The model under review builds one solid part; all positions refer to its coordinate system, in mm. Coordinates: 2 decimals unless noted, no trailing zeros. Write each loop counter-clockwise with the first axis right and the second up, starting at its lowest first coordinate (ties: lowest second). Pieces come first, ordered by that corner, then holes. Notation, with made-up numbers: (41, -11) -> (69, -11) arc R12 ccw to (69, 11) -> close; hole circle Ø11 at (76, -21). An arc over 180 degrees is marked (long way). Put each result on its own line as item: value. Start each with the question number.
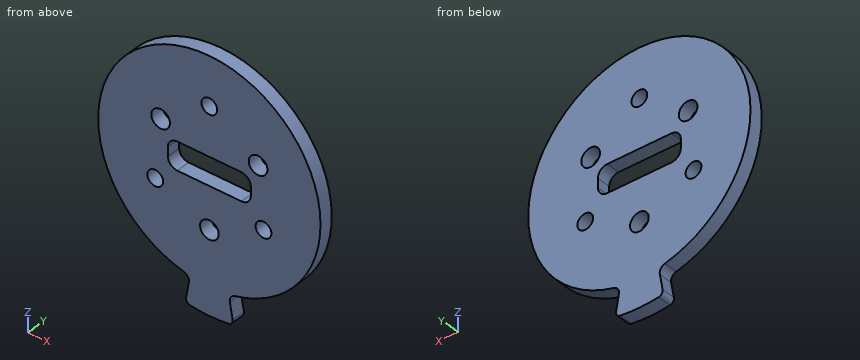
from build123d import *

# Parameters (mm, degrees)
SKETCH_1_R          = 30
EXTRUDE_1_DEPTH     = 3
SKETCH_2_R          = 1.7
SKETCH_2_R_2        = 2.015
CUT_EXTRUDE_1_DEPTH = 3
CUT_EXTRUDE_START   = -3
CUT_EXTRUDE_2_DEPTH = 3
FILLET_1_R          = 1.5
FILLET_2_R          = 1
SKETCH_4_W          = 17.9
SKETCH_4_H          = 6.05
CUT_EXTRUDE_3_DEPTH = 10
FILLET_3_R          = 2.03


with BuildPart() as part:
    # 草图1 → 凸台-拉伸1 (new body)
    with BuildSketch(Plane(origin=(0, 0, 0), x_dir=(1, 0, 0), z_dir=(0, 1, 0))):
        with Locations(Location((0, 0, 0), (0, 0, 270))):
            Circle(SKETCH_1_R)
    extrude(amount=EXTRUDE_1_DEPTH)

    # 草图2 → 切除-拉伸1 (cut)
    with BuildSketch(Plane(origin=(0, 3, 0), x_dir=(1, 0, 0), z_dir=(0, 1, 0))):
        with Locations(Location((0, -13.5, 0), (0, 0, 270))):
            Circle(SKETCH_2_R)
        with Locations(Location((-11.691342951, 6.75, 0), (0, 0, 270))):
            Circle(SKETCH_2_R)
        with Locations(Location((11.691342951, 6.75, 0), (0, 0, 270))):
            Circle(SKETCH_2_R)
        with Locations(Location((10.522208656, -6.075, 0), (0, 0, 270))):
            Circle(SKETCH_2_R_2)
        with Locations(Location((-10.522208656, -6.075, 0), (0, 0, 270))):
            Circle(SKETCH_2_R_2)
        with Locations(Location((0, 12.15, 0), (0, 0, 270))):
            Circle(SKETCH_2_R_2)
    extrude(amount=-CUT_EXTRUDE_1_DEPTH, mode=Mode.SUBTRACT)

    # 草图3 → 切除-拉伸2 (cut)
    with BuildSketch(Plane(origin=(0, 3, 0), x_dir=(1, 0, 0), z_dir=(0, 1, 0)).offset(CUT_EXTRUDE_START)):
        with BuildLine():
            Line((-5.20944533, 29.54423259), (-4.167556264, 23.635386072))
            ThreePointArc((-4.167556264, 23.635386072), (0, -24), (4.167556264, 23.635386072))
            Line((4.167556264, 23.635386072), (5.20944533, 29.54423259))
            ThreePointArc((5.20944533, 29.54423259), (0, -30), (-5.20944533, 29.54423259))
        make_face()
    extrude(amount=CUT_EXTRUDE_2_DEPTH, mode=Mode.SUBTRACT)

    # 圆角1
    fillet_1_edges = [part.edges().sort_by_distance(p)[0] for p in [
        (-4.167556264, 1.5, -23.635386072),
        (4.167556264, 1.5, -23.635386072),
    ]]
    fillet(fillet_1_edges, radius=FILLET_1_R)

    # 圆角2
    fillet_2_edges = [part.edges().sort_by_distance(p)[0] for p in [
        (5.20944533, 1.5, -29.54423259),
        (-5.20944533, 1.5, -29.54423259),
    ]]
    fillet(fillet_2_edges, radius=FILLET_2_R)

    # 草图4 → 切除-拉伸3 (cut)
    with BuildSketch(Plane(origin=(0, 3, 0), x_dir=(1, 0, 0), z_dir=(0, 1, 0))):
        Rectangle(SKETCH_4_W, SKETCH_4_H)
    extrude(amount=-CUT_EXTRUDE_3_DEPTH, mode=Mode.SUBTRACT)

    # 圆角3
    fillet_3_edges = [part.edges().sort_by_distance(p)[0] for p in [
        (8.95, 1.5, -3.025),
        (8.95, 1.5, 3.025),
        (-8.95, 1.5, 3.025),
        (-8.95, 1.5, -3.025),
    ]]
    fillet(fillet_3_edges, radius=FILLET_3_R)


solid = part.part
1. Consider section B-B on z = 0. State the section outline as (x, y) points, then the cut area to 3 significant figures.
2. Consider section D-D on y = 2.45. State the section outline as (x, z) points (3 decimals).
3. Consider section A-A on x = 0. State the section outline as (y, z) points (3 decimals).
4. Consider section C-C on z = -6.75. State the section outline as (x, y) points, then the cut area to 3 significant figures.
5. Insertion check: P1, Ø1.5, axis at x = -1, y = 1, coming from the +Z side. The pin has a flat end and moves straight along its axis. Give the tip position at first contact, or say it passes through.
6. Wall thickness on line 1 (Z direction, x = -12, y = 1); line 2 (Z direction, x = -11, y = 1.65); line 3 (Z direction, x = 1.5, y = 1.8) (3 decimals): over which ranges is each line inside the solid? List them lowest first. Write a range as from..to.
Output values:
1. outline: (-24, 0) -> (-8.95, 0) -> (-8.95, 3) -> (-24, 3) -> close; (8.95, 0) -> (24, 0) -> (24, 3) -> (8.95, 3) -> close
1. area: 90.3 mm^2
2. outline: (-5.551, -23.349) arc R1.5 cw to (-4.42, -25.069) -> (-5.033, -28.542) arc R1 ccw to (-4.188, -29.706) arc R30 ccw to (4.188, -29.706) arc R1 ccw to (5.033, -28.542) -> (4.42, -25.069) arc R1.5 cw to (5.551, -23.349) arc R24 ccw (long way) to start; hole circle Ø3.4 at (-11.691, -6.75); hole circle Ø4.03 at (-10.522, 6.075); hole (-8.95, -0.995) arc R2.03 ccw to (-6.92, -3.025) -> (6.92, -3.025) arc R2.03 ccw to (8.95, -0.995) -> (8.95, 0.995) arc R2.03 ccw to (6.92, 3.025) -> (-6.92, 3.025) arc R2.03 ccw to (-8.95, 0.995) -> close; hole circle Ø4.03 at (0, -12.15); hole circle Ø3.4 at (0, 13.5); hole circle Ø4.03 at (10.522, 6.075); hole circle Ø3.4 at (11.691, -6.75)
3. outline: (0, -30) -> (3, -30) -> (3, -14.165) -> (0, -14.165) -> close; (0, -10.135) -> (3, -10.135) -> (3, -3.025) -> (0, -3.025) -> close; (0, 3.025) -> (3, 3.025) -> (3, 11.8) -> (0, 11.8) -> close; (0, 15.2) -> (3, 15.2) -> (3, 24) -> (0, 24) -> close
4. outline: (-23.03, 0) -> (-13.39, 0) -> (-13.39, 3) -> (-23.03, 3) -> close; (-9.99, 0) -> (9.99, 0) -> (9.99, 3) -> (-9.99, 3) -> close; (13.39, 0) -> (23.03, 0) -> (23.03, 3) -> (13.39, 3) -> close
4. area: 118 mm^2
5. P1: stops at z = 24
6. line 1: z = -20.78..-8.42, -5.08..4.71, 7.44..20.78
6. line 2: z = -21.33..-8.3, -5.2..4.12, 8.03..21.33
6. line 3: z = -29.962..-13.495, -10.805..-3.025, 3.025..12.7, 14.3..23.953
